Here's how the part is built. I have some questions about the finished solid (model axes, mm). Face numbers are marked on the shaded views. Coordinates: 2 decimals unless noted, no trailing zeros. Write each loop counter-clockwise with the first axis right and the second up, starting at its lowest first coordinate (ties: lowest second). Pieces come first, ordered by that corner, then holes. Notation, with made-up numbers: (59.25, -19.75) -> (103.25, -19.75) arc R14 ccw to (103.25, -11.75) -> close; hole circle Ø8 at (31.25, 25.25). An arc over 180 degrees is marked (long way). Put each result on its own line as item: value.
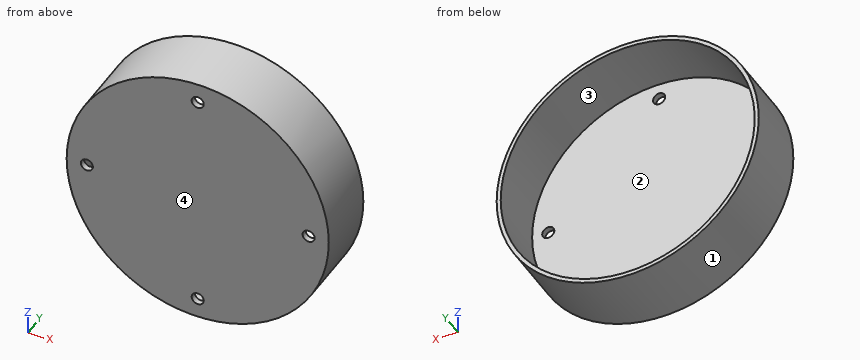
```python
from build123d import *

# Parameters (mm, degrees)
SKETCH1_R           = 65
BOSS_EXTRUDE1_DEPTH = 3
SKETCH2_R           = 3
CUT_EXTRUDE1_DEPTH  = 4
CIRPATTERN1_COUNT   = 4
SKETCH3_R           = 65
SKETCH3_R_2         = 63
BOSS_EXTRUDE2_DEPTH = 30


with BuildPart() as part:
    # Sketch1 → Boss-Extrude1 (new body)
    with BuildSketch(Plane(origin=(0, 0, 0), x_dir=(1, 0, 0), z_dir=(0, 1, 0))):
        Circle(SKETCH1_R)
    extrude(amount=BOSS_EXTRUDE1_DEPTH)

    # Sketch2 → Cut-Extrude1 (cut, through all)
    with BuildSketch(Plane(origin=(0, 3, 0), x_dir=(1, 0, 0), z_dir=(0, 1, 0))):
        with Locations((0, 55)):
            Circle(SKETCH2_R)
    cut_extrude1 = extrude(amount=-CUT_EXTRUDE1_DEPTH, mode=Mode.SUBTRACT)

    # CirPattern1: Cut-Extrude1 ×4 about axis
    cirpattern1_axis = Axis((0, 0, 0), (0, 1, 0))
    for i in range(1, CIRPATTERN1_COUNT):
        add(cut_extrude1.rotate(cirpattern1_axis, i * 360 / CIRPATTERN1_COUNT), mode=Mode.SUBTRACT)

    # Sketch3 → Boss-Extrude2 (add)
    with BuildSketch(Plane(origin=(0, 3, 0), x_dir=(1, 0, 0), z_dir=(0, 1, 0))):
        Circle(SKETCH3_R)
        Circle(SKETCH3_R_2, mode=Mode.SUBTRACT)
    extrude(amount=BOSS_EXTRUDE2_DEPTH)


solid = part.part
```
Item 1: Imagine slicing it at D-D on x = 55. Write out the boundary of the cut face in (y, z).
Output:
outline: (0, -34.64) -> (33, -34.64) -> (33, -30.72) -> (3, -30.72) -> (3, -3) -> (0, -3) -> close; (0, 3) -> (3, 3) -> (3, 30.72) -> (33, 30.72) -> (33, 34.64) -> (0, 34.64) -> close
Item 2: Please list where these lines run through material, in increasing order: line 1 along Z through (x, y) = (0, 1); line 2 along Y through (x, z) = (-37, 43); line 3 along Z through (x, y) = (47, 30). Write a range as from..to.
Output:
line 1: z = -65..-58, -52..52, 58..65
line 2: y = 0..3
line 3: z = -44.9..-41.95, 41.95..44.9
Item 3: For P1, Ø3, axis at x = -48.5, z = -1, coming from the +Y side; P2, Ø4, axis at x = -4, y = 8.5, coming from the +Z side; P3, Ø1, axis at x = -22, y = 17.5, coming from the +Z side, each with a flat end and sliding along its axis, tell me the tip position at first contact or that it passes through.
Output:
P1: stops at y = 3
P2: stops at z = 64.97
P3: stops at z = 61.34
Item 4: Imagine slicing it at B-B on z = 0. Write out the boundary of the cut face in (x, y).
Output:
outline: (-65, 0) -> (-58, 0) -> (-58, 3) -> (-63, 3) -> (-63, 33) -> (-65, 33) -> close; (-52, 0) -> (52, 0) -> (52, 3) -> (-52, 3) -> close; (58, 0) -> (65, 0) -> (65, 33) -> (63, 33) -> (63, 3) -> (58, 3) -> close
Item 5: Imagine slicing it at C-C on z = 55. Write out the boundary of the cut face in (x, y), then the cut area to 3 significant figures.
Output:
outline: (-34.64, 0) -> (-3, 0) -> (-3, 3) -> (-30.72, 3) -> (-30.72, 33) -> (-34.64, 33) -> close; (3, 0) -> (34.64, 0) -> (34.64, 33) -> (30.72, 33) -> (30.72, 3) -> (3, 3) -> close
area: 425 mm²
Item 6: If we mould it in two halves opening along Z, with no side actions, what happens to the marked faces 1, 2, 3 and 4? For each: released by +Z, released by -Z, zero draft, split by the parting line, or undercut.
Output:
face 1: split by the parting line
face 2: undercut
face 3: undercut
face 4: zero draft
Item 7: Imagine slicing it at A-A on x = 0. Write out the boundary of the cut face in (y, z), then the cut area to 3 significant figures.
Output:
outline: (0, -65) -> (33, -65) -> (33, -63) -> (3, -63) -> (3, -58) -> (0, -58) -> close; (0, -52) -> (3, -52) -> (3, 52) -> (0, 52) -> close; (0, 58) -> (3, 58) -> (3, 63) -> (33, 63) -> (33, 65) -> (0, 65) -> close
area: 474 mm²
